Part model, mm, in its own coordinate system. A direction names the side the tool comes from. Round coordinates to 2 decimals unless told otherwise and drop trailing zeros. Order: outer loops, then holes, each group sorted by start corner. A loop starts at its lowest first (then second) coordinate and runs counter-clockwise, first axis right, second up. Notation, with made-up numbers: M -37,0.25 L 9,0.25 A19 ccw 9,17.25 Z; hole C -15,24 d5. An arc over 180 degrees is marked long. One line per question, with ' | ' between items.
from build123d import *

# Parameters (mm, degrees)
EXTRUDE_1_DEPTH     = 3.9
SKETCH_3_R          = 3
EXTRUDE_3_DEPTH     = 5
CHAMFER_1_SIZE      = 0.75
SKETCH_2_OUTSIDE_W  = 15.536
SKETCH_2_OUTSIDE_H  = 17.084
SKETCH_2_OUTSIDE_R  = 4.5
CUT_EXTRUDE_1_DEPTH = 0.26
FILLET_1_R          = 0.1


with BuildPart() as part:
    # Sketch 1 → Extrude 1 (new body)
    with BuildSketch(Plane.XY):
        Polygon((0, 5.773502692), (-5, 2.886751346), (-5, -2.886751346), (0, -5.773502692), (5, -2.886751346), (5, 2.886751346), align=None)
    extrude(amount=EXTRUDE_1_DEPTH)

    # Sketch 3 → Extrude 3 (add)
    with BuildSketch(Plane.XY):
        Circle(SKETCH_3_R)
    extrude(amount=-EXTRUDE_3_DEPTH)

    # Sketch 4 → Cut-Revolve 1 (revolve, cut)
    with BuildSketch(Plane(origin=(0, 0, 0), x_dir=(0, 0, -1), z_dir=(1, 0, 0)), mode=Mode.PRIVATE) as cut_revolve_1_sk:
        Polygon((-3.9, 20), (-3.9, 4), (0.387187079, 20), align=None)
    revolve(cut_revolve_1_sk.sketch.rotate(Axis((0, 0, -2.242017917), (0, 0, 1)), 90), axis=Axis((0, 0, -2.242017917), (0, 0, 1)), mode=Mode.SUBTRACT)

    # Chamfer 1
    chamfer_1_edges = [part.edges().sort_by_distance(p)[0] for p in [
        (-3, 0, -5),
    ]]
    chamfer(chamfer_1_edges, length=CHAMFER_1_SIZE)

    # Sketch 2 outside → Cut-Extrude 1 (cut)
    with BuildSketch(Plane.XY):
        Rectangle(SKETCH_2_OUTSIDE_W, SKETCH_2_OUTSIDE_H)
        Circle(SKETCH_2_OUTSIDE_R, mode=Mode.SUBTRACT)
    extrude(amount=CUT_EXTRUDE_1_DEPTH, mode=Mode.SUBTRACT)

    # Fillet 1
    fillet_1_edges = [part.edges().sort_by_distance(p)[0] for p in [
        (-3, 0, 0),
    ]]
    fillet(fillet_1_edges, radius=FILLET_1_R)


solid = part.part
1) Saw through at C-C (z = -3.25). List the corners of the cut face in (x, y), plus the area to 3 significant figures.
The answers:
outline: C 0,0 d6 | area: 28.3 mm²
2) Drop flat-ended pins along their axis: pin 1 (3 mm diameter, centred on x = -2, z = 0.5, fed in from +Y); pin 2 (4 mm diameter, centred on x = 3.5, y = 1.5, fed in from -Z); pin 3 (3 mm diameter, centred on x = 0, y = -4, fed in from -Z); pin 4 (2 mm diameter, centred on x = 3.5, z = -3.5, fed in from +Y). Give the stop position or say it passes through.
The answers:
pin 1: stops at y = 5.48 | pin 2: stops at z = -5 | pin 3: stops at z = -4.75 | pin 4: stops at y = 1.66
3) Probe line 1 (Z direction, x = -1.75, y = 2.75); line 2 (X direction, y = 1.5, z = -0.75); line 3 (X direction, y = -1, z = -0.5). List the from-to ranges inside material, lowest first. Write a range as [from, to].
The answers:
line 1: z = [0, 3.9] | line 2: x = [-2.6, 2.6] | line 3: x = [-2.83, 2.83]
4) Saw through at B-B (z = 2). List the corners of the cut face in (x, y), plus the area to 3 significant figures.
The answers:
outline: M -5,-2.89 L 0,-5.77 L 5,-2.89 L 5,2.89 L 0,5.77 L -5,2.89 Z | area: 86.6 mm²
5) Saw through at A-A (y = 0). List the corners of the cut face in (x, z).
The answers:
outline: M -5,0.26 L -4.5,0.26 L -4.5,0 L -3.1,0 A0.1 cw -3,-0.1 L -3,-4.25 L -2.25,-5 L 2.25,-5 L 3,-4.25 L 3,-0.1 A0.1 cw 3.1,0 L 4.5,0 L 4.5,0.26 L 5,0.26 L 5,3.63 L 4,3.9 L -4,3.9 L -5,3.63 Z
6) Which spindle directions (+Z, -Z, +X, -X, +Y, -Y) get a long thin tool onto all of the face, cutting with end or side? Do faces 1 (the face through (0, -5, 0.26)), 2 (the face through (0, 0, -5)). Say none if no direction does.
The answers:
face 1: -Z | face 2: -Z, +X, -X, +Y, -Y
